Check sheet for the drawn part. Datum: minimum x, y, z corner. Units: mm. A direction names the side the tool comes from. Give positions to 0.01 mm unless a question says otherwise; leave off trailing zeros. Order: outer loops, then holes, each group sorted by start corner. A loop starts at its lowest first (then second) coordinate and runs counter-clockwise, first axis right, second up. Notation, with made-up numbers: (-7.5, 31) -> (43.5, 31) arc R29 cw to (43.5, 68) -> close; hole circle Ø10 at (3.5, -34). An arc over 180 degrees is marked (long way). Return JSON: item names as keys, results as strings. Group by question number.
(1) Thickness scan on line 1 along Y through (x, z) = (3.2, 2.25); line 2 along Y through (x, z) = (6, 4.75); line 3 along Y through (x, z) = (18.25, 3.25). Record the ranges inside material, lowest first.
(2) Cross-section at A-A on x = 11. Enter the section's corners in (y, z).
(3) Release check for a two-part mould opening along Y. For the marked faces 4, 5 and 6 record: pulls with the +Y half, pulls with the -Y half, needs draft (parallel to the pull), parting line crosses it, or undercut.
(4) Cross-section at D-D on z = 2.5. Enter the section's corners in (x, y).
(5) Tool access check on the marked faces 1, 2 and 3. Record the directions out of +Z, -Z, +X, -X, +Y, -Y that give a thin tool (end or side, any length) a straight path to the whole face; none if there is none.
(6) Cross-section at B-B on y = 43.65. Enter the section's corners in (x, z).
(7) Depth check by flat-ended pin: pin 1 Ø1.7 at (x, y) = (18.8, 43.65) entering from -Z; pin 2 Ø1.9 at (y, z) = (21.5, 4) entering from +X. Enter the tip coordinate at first touch or a pass-through.
(8) Cross-section at C-C on x = 18.8. Enter the section's corners in (y, z).
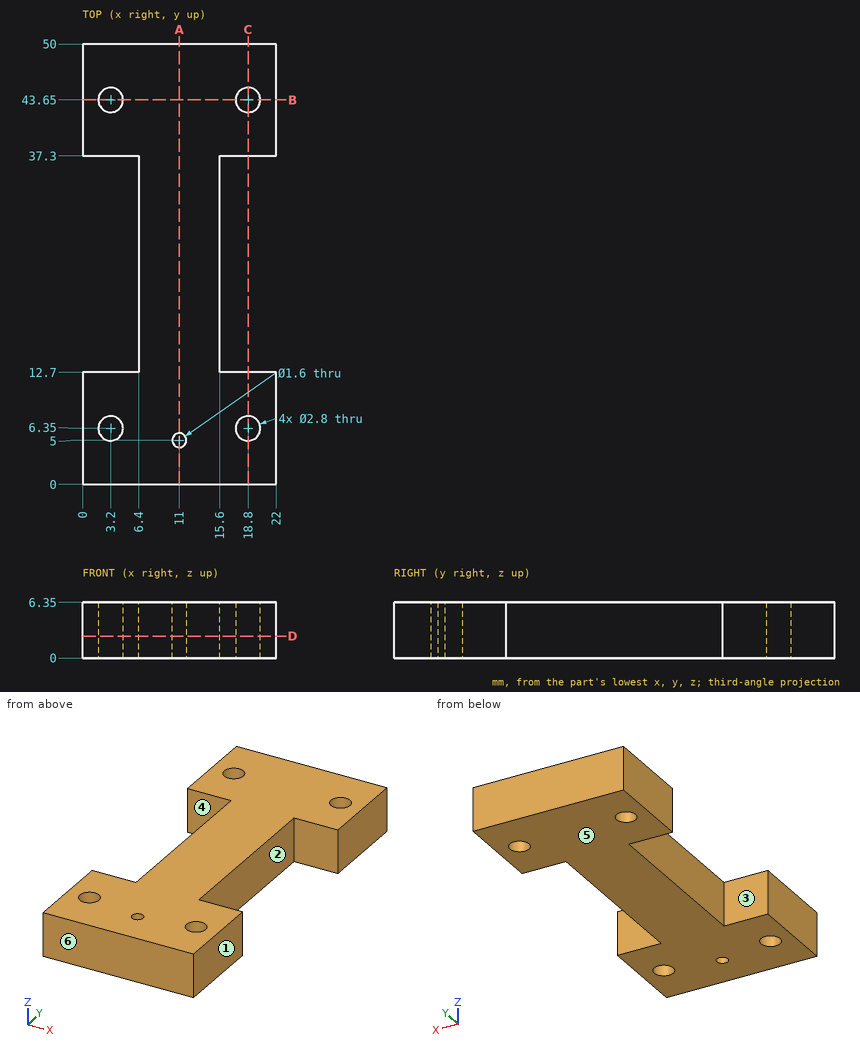
Verdict:
{
 "1": {"line 1": "0 to 4.95, 7.75 to 12.7, 37.3 to 42.25, 45.05 to 50", "line 2": "0 to 12.7, 37.3 to 50", "line 3": "0 to 5.06, 7.64 to 12.7, 37.3 to 42.36, 44.94 to 50"},
 "2": {"outline": "(0, 0) -> (4.2, 0) -> (4.2, 6.35) -> (0, 6.35) -> close; (5.8, 0) -> (50, 0) -> (50, 6.35) -> (5.8, 6.35) -> close"},
 "3": {"face 4": "undercut", "face 5": "needs draft", "face 6": "pulls with the -Y half"},
 "4": {"outline": "(0, 0) -> (22, 0) -> (22, 12.7) -> (15.6, 12.7) -> (15.6, 37.3) -> (22, 37.3) -> (22, 50) -> (0, 50) -> (0, 37.3) -> (6.4, 37.3) -> (6.4, 12.7) -> (0, 12.7) -> close; hole circle Ø2.8 at (3.2, 6.35); hole circle Ø2.8 at (3.2, 43.65); hole circle Ø1.6 at (11, 5); hole circle Ø2.8 at (18.8, 6.35); hole circle Ø2.8 at (18.8, 43.65)"},
 "5": {"face 1": "+Z, -Z, +X, +Y, -Y", "face 2": "+Z, -Z, +X", "face 3": "+Z, -Z, -X"},
 "6": {"outline": "(0, 0) -> (1.8, 0) -> (1.8, 6.35) -> (0, 6.35) -> close; (4.6, 0) -> (17.4, 0) -> (17.4, 6.35) -> (4.6, 6.35) -> close; (20.2, 0) -> (22, 0) -> (22, 6.35) -> (20.2, 6.35) -> close"},
 "7": {"pin 1": "through", "pin 2": "x = 15.6"},
 "8": {"outline": "(0, 0) -> (4.95, 0) -> (4.95, 6.35) -> (0, 6.35) -> close; (7.75, 0) -> (12.7, 0) -> (12.7, 6.35) -> (7.75, 6.35) -> close; (37.3, 0) -> (42.25, 0) -> (42.25, 6.35) -> (37.3, 6.35) -> close; (45.05, 0) -> (50, 0) -> (50, 6.35) -> (45.05, 6.35) -> close"}
}
